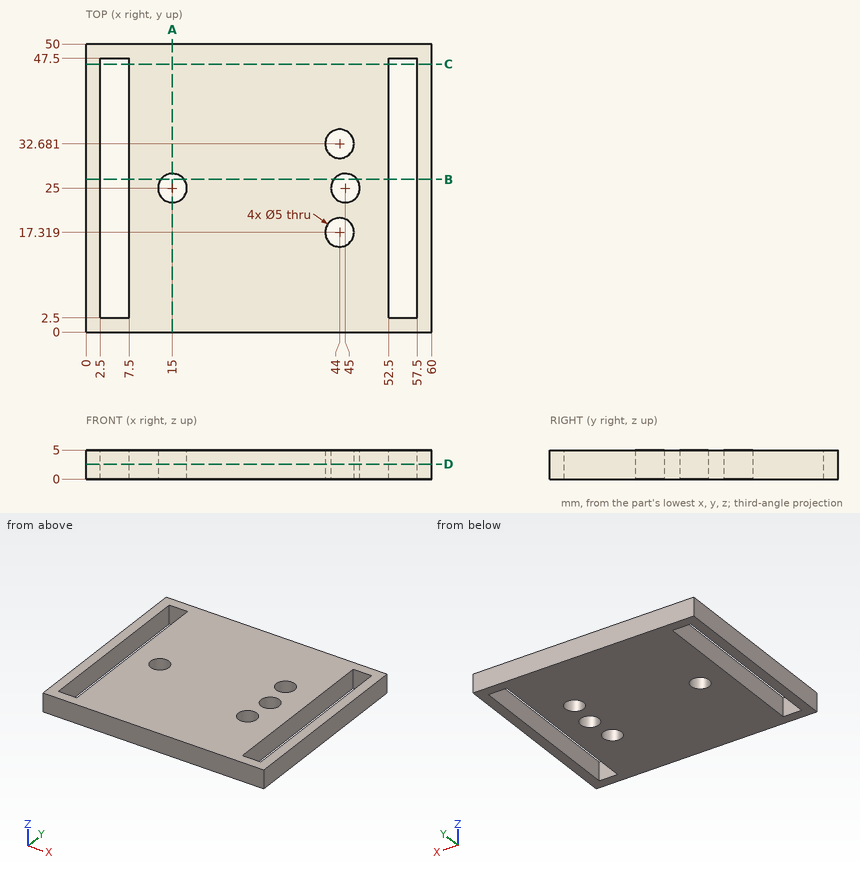
Here's the drawing with two shaded views (mm, measured from the low corner). I have some questions. Give positions to 0.01 mm unless a question says otherwise; leave off trailing zeros. Write each loop counter-clockwise with the first axis right and the second up, starting at its lowest first coordinate (ties: lowest second). Pieces come first, ordered by that corner, then holes. Notation, with made-up numbers: (-20, 12.5) -> (-12, 12.5) arc R17 ccw to (-12, 44.5) -> close; hole circle Ø4 at (69.5, -15). An arc over 180 degrees is marked (long way). Answer as a JSON object with one key per item and string values. Group by question number.
Item 1: Suppose I cut it at A-A (x = 15). Please give me the cut outline in (y, z), plus the area to 3 significant figures.
Item 2: Please list where these lines run through material, in increasing order: line 1 (X direction, y = 14, z = 2.8); line 2 (Y direction, x = 44, z = 3.75); line 3 (Y direction, x = 15, z = 3.5). Write a range as [from, to].
Item 3: I'm going to push a flat-ended pin straight in: P1, Ø4.5, axis at x = 44, y = 32.68, coming from the -Z side. Where does the tip first touch, or does it pass through?
Item 4: Suppose I cut it at D-D (z = 2.6). Please give me the cut outline in (x, y), plus the area to 3 significant figures.
Item 5: Suppose I cut it at C-C (y = 46.5). Please give me the cut outline in (x, z).
Item 6: Suppose I cut it at B-B (y = 26.5). Please give me the cut outline in (x, z), plus the area to 3 significant figures.
Findings:
{
 "1": {"outline": "(0, 0) -> (22.5, 0) -> (22.5, 5) -> (0, 5) -> close; (27.5, 0) -> (50, 0) -> (50, 5) -> (27.5, 5) -> close", "area": "225 mm²"},
 "2": {"line 1": "x = [0, 2.5], [7.5, 52.5], [57.5, 60]", "line 2": "y = [0, 14.82], [19.82, 22.71], [27.29, 30.18], [35.18, 50]", "line 3": "y = [0, 22.5], [27.5, 50]"},
 "3": {"P1": "passes through"},
 "4": {"outline": "(0, 0) -> (60, 0) -> (60, 50) -> (0, 50) -> close; hole (2.5, 2.5) -> (7.5, 2.5) -> (7.5, 47.5) -> (2.5, 47.5) -> close; hole circle Ø5 at (15, 25); hole circle Ø5 at (44, 17.32); hole circle Ø5 at (44, 32.68); hole circle Ø5 at (45, 25); hole (52.5, 2.5) -> (57.5, 2.5) -> (57.5, 47.5) -> (52.5, 47.5) -> close", "area": "2,470 mm²"},
 "5": {"outline": "(0, 0) -> (2.5, 0) -> (2.5, 5) -> (0, 5) -> close; (7.5, 0) -> (52.5, 0) -> (52.5, 5) -> (7.5, 5) -> close; (57.5, 0) -> (60, 0) -> (60, 5) -> (57.5, 5) -> close"},
 "6": {"outline": "(0, 0) -> (2.5, 0) -> (2.5, 5) -> (0, 5) -> close; (7.5, 0) -> (13, 0) -> (13, 5) -> (7.5, 5) -> close; (17, 0) -> (43, 0) -> (43, 5) -> (17, 5) -> close; (47, 0) -> (52.5, 0) -> (52.5, 5) -> (47, 5) -> close; (57.5, 0) -> (60, 0) -> (60, 5) -> (57.5, 5) -> close", "area": "210 mm²"}
}
